Work out the finished part from the listing and answer in its coordinate system (mm). A direction names the side the tool comes from. Coordinates: 2 decimals unless noted, no trailing zeros. Order: outer loops, then holes, each group sorted by start corner. A loop starts at its lowest first (then second) coordinate and runs counter-clockwise, first axis right, second up. Notation, with made-up numbers: (89, 49.25) -> (93, 49.25) arc R29 cw to (93, 75.25) -> close; hole circle Ø4 at (7.5, 67). An arc over 180 degrees is marked (long way). Write item = value, one per line. Start each with the question number.
Q1. For a pull along Y with two mould halves and no side action, classify faces 3 (the cylindrical face through (33.734, -31.273, 10.846)), 4 (the flat face through (-1, 1, 2)), 5 (the cylindrical face through (42.445, 13.367, 12.14)), 6 (the cylindrical face through (-45.992, 0.847, 3.513)) as +Y half, -Y half, draft (parallel to the pull), parting line (faces both ways), or undercut.
Q2. The part is cut by section C-C, the plane z = 13.75. Count the separate pieces of the cut face and the enclosed holes in it, plus the area to 3 significant figures.
Q3. Which of the six approach directions +Z, -Z, +X, -X, +Y, -Y give full straight-line access (tool end or side, diameter ignored) to faces 1 (the cylindrical face through (-0.54, -53.44, 10.85)), 2 (the cylindrical face through (-45, -0.1, 4.5))?
Q4. The part is cut by section B-B, the plane y = 0. Determine the outline of the cut face in (x, z), plus the area to 4 significant figures.
Q5. The part is cut by section A-A, the plane x = 0. Determine the outline of the cut face in (y, z).
Q6. Straight lines are drawn through the part: L1, parallel to X at y = 0, z = 8.5; L2, parallel to Z at x = -37, y = 9; L3, parallel to X at y = 7.5, z = 4.25. For each, find the intervals that lie inside material, in ascending order. Write a range as from..to.
Q7. Flat-ended cylindrical pins translate along their axes: pin 1 (10 mm diameter, centred on x = -7, y = -25.5, fed in from -Z); pin 2 (5 mm diameter, centred on y = 17.5, z = 6, fed in from -X); pin 3 (0.9 mm diameter, centred on x = 36.5, z = 19.5, fed in from -Y); pin 4 (4 mm diameter, centred on y = 4, z = 3, fed in from +X). Find the tip coordinate at first contact, or state that the pin passes through.
Q8. The part is cut by section D-D, the plane x = 33. Determine the outline of the cut face in (y, z).
```python
from build123d import *

# Parameters (mm, degrees)
F0_R     = 2.5
F1_DEPTH = 22
F3_W     = 52
F3_H     = 5.5
F4_DEPTH = 115.138352
F5_R     = 44.5
F6_DEPTH = 20
F2_R     = 17.5
F7_DEPTH = 60.93917
F8_R     = 5


with BuildPart() as f1:
    # F0 (on Top) → F1 (new body)
    with BuildSketch(Plane.XY):
        with BuildLine():
            Line((45.384134, -7.502026), (45.385261, -7.495206))
            ThreePointArc((45.385261, -7.495206), (36.922436, 27.435993), (5.918638, 45.617647))
            ThreePointArc((5.918638, 45.617647), (0, 59), (-5.918638, 45.617647))
            ThreePointArc((-5.918638, 45.617647), (-46, 0), (-5.918638, -45.617647))
            ThreePointArc((-5.918638, -45.617647), (0, -59), (5.918638, -45.617647))
            ThreePointArc((5.918638, -45.617647), (31.956122, -33.087857), (45.384134, -7.502026))
        make_face()
        with Locations((0, -51)):
            Circle(F0_R, mode=Mode.SUBTRACT)
        with Locations((0, 51)):
            Circle(F0_R, mode=Mode.SUBTRACT)
    extrude(amount=F1_DEPTH)

    # F3 (on Right) → F4 (cut)
    with BuildSketch(Plane.YZ):
        with Locations((0.416768, 19.25)):
            Rectangle(F3_W, F3_H)
    extrude(amount=F4_DEPTH, mode=Mode.SUBTRACT)

    # F5 (on face) → F6 (cut)
    with BuildSketch(Plane.XY.offset(22)):
        Circle(F5_R)
    extrude(amount=-F6_DEPTH, mode=Mode.SUBTRACT)

    # F2 (on Right) → F7 (cut)
    with BuildSketch(Plane.YZ):
        with Locations((0, 22)):
            Circle(F2_R)
    extrude(amount=-F7_DEPTH, mode=Mode.SUBTRACT)

    # F8
    f8_edges = [f1.edges().sort_by_distance(p)[0] for p in [
        (-5.918638, -45.617647, 11),
        (5.918638, -45.617647, 11),
        (5.918638, 45.617647, 11),
        (-5.918638, 45.617647, 11),
    ]]
    fillet(f8_edges, radius=F8_R)


solid = f1.part
```
Model answer:
q1.face_3 = -Y half
q1.face_4 = undercut
q1.face_5 = undercut
q1.face_6 = parting line
q2.separate_pieces = 1
q2.enclosed_holes = 2
q2.area = 719 mm2
q3.face_1 = +Z, -Z
q3.face_2 = +Z, -X
q4.outline = (-46, 0) -> (46, 0) -> (46, 16.5) -> (44.5, 16.5) -> (44.5, 2) -> (-44.5, 2) -> (-44.5, 4.5) -> (-46, 4.5) -> close
q4.area = 209.5 mm2
q5.outline = (-59, 0) -> (-53.5, 0) -> (-53.5, 22) -> (-59, 22) -> close; (-48.5, 0) -> (48.5, 0) -> (48.5, 22) -> (44.5, 22) -> (44.5, 2) -> (-44.5, 2) -> (-44.5, 22) -> (-48.5, 22) -> close; (53.5, 0) -> (59, 0) -> (59, 22) -> (53.5, 22) -> close
q6.L1 = 44.5..46
q6.L2 = 0..2
q6.L3 = -45.38..-43.86, 43.86..45.38
q7.pin_1 = 0
q7.pin_2 = -43.49
q7.pin_3 = -28.57
q7.pin_4 = 45.96
q8.outline = (-32.05, 0) -> (32.05, 0) -> (32.05, 22) -> (29.85, 22) -> (29.85, 2) -> (-29.85, 2) -> (-29.85, 22) -> (-32.05, 22) -> close
